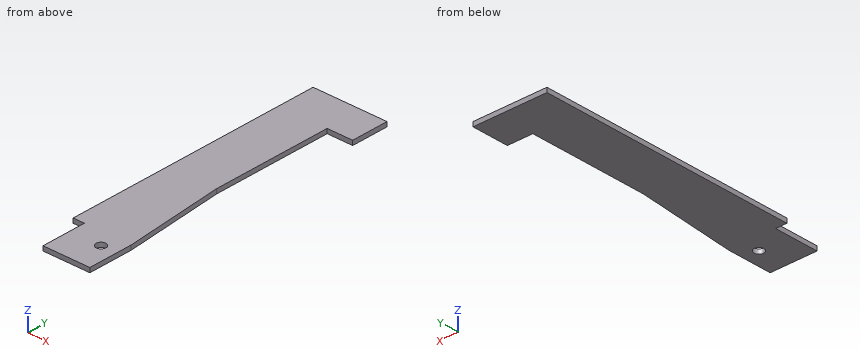
```python
from build123d import *

# Parameters (mm, degrees)
EXTRUDE_2_DEPTH     = 1
SKETCH_1_5_W        = 5.5
SKETCH_1_5_H        = 10
SKETCH_1_5_W_2      = 4.949873967
SKETCH_1_5_R        = 1.1
EXTRUDE_3_DEPTH     = 1
SKETCH_3_W          = 3
SKETCH_3_H          = 58
CUT_EXTRUDE_1_DEPTH = 10


with BuildPart() as part:
    # 草图1 → 凸台-拉伸2 (new body)
    with BuildSketch(Plane.XY):
        Polygon((-5.588804059, 13.118731113), (-5.588804059, -12.701827406), (-5.588804059, -40.201827406), (-0.088804059, -40.201827406), (5.411195941, -40.201827406), (10.361069908, -40.201827406), (8.211195941, -17.197725842), (8.211195941, 9.5), (13.911195941, 9.5), (13.911195941, 12.5), (13.911195941, 17.798172594), (-5.588804059, 17.798172594), align=None)
    extrude(amount=EXTRUDE_2_DEPTH)

    # 草图1<5> → 凸台-拉伸3 (add)
    # profile 1 of 3: a face of its own
    with BuildSketch(Plane.XY):
        Polygon((-5.588804059, 13.118731113), (-5.588804059, -12.701827406), (-5.588804059, -40.201827406), (-0.088804059, -40.201827406), (5.411195941, -40.201827406), (10.361069908, -40.201827406), (8.211195941, -17.197725842), (8.211195941, 9.5), (13.911195941, 9.5), (13.911195941, 12.5), (13.911195941, 17.798172594), (-5.588804059, 17.798172594), align=None)
    # profile 2 of 3: a face of its own
    with BuildSketch(Plane.XY):
        with Locations((2.661195941, -45.201827406)):
            Rectangle(SKETCH_1_5_W, SKETCH_1_5_H)
    # profile 3 of 3: a face of its own
    with BuildSketch(Plane.XY):
        with Locations((7.886132925, -45.201827406)):
            Rectangle(SKETCH_1_5_W_2, SKETCH_1_5_H)
        with Locations((6.861069908, -43.701827406)):
            Circle(SKETCH_1_5_R, mode=Mode.SUBTRACT)
    extrude(amount=EXTRUDE_3_DEPTH)

    # 草图3 → 切除-拉伸1 (cut)
    with BuildSketch(Plane.XY.offset(1)):
        with Locations((-4.088804059, -11.201827406)):
            Rectangle(SKETCH_3_W, SKETCH_3_H)
    extrude(amount=-CUT_EXTRUDE_1_DEPTH, mode=Mode.SUBTRACT)


solid = part.part
```
Design review of the part built by this model. Coordinates are the model's own, in mm. Round coordinates to 2 decimals unless told otherwise and drop trailing zeros. Write each loop counter-clockwise with the first axis right and the second up, starting at its lowest first coordinate (ties: lowest second). Pieces come first, ordered by that corner, then holes. Notation, with made-up numbers: (78.5, 67.5) -> (106.5, 67.5) arc R25 ccw to (106.5, 93.5) -> close; hole circle Ø4 at (8.25, 49). An arc over 180 degrees is marked (long way). Answer in a Markdown table with one row per item.
Q1. Take a section at C-C, the plane y = -41.5. State the section outline as (x, z) points.
The answers:
| item | result |
|---|---|
| outline | (-0.09, 0) -> (10.36, 0) -> (10.36, 1) -> (-0.09, 1) -> close |
Q2. Clearance check with flat-ended pins moving along their axes: pin 1 Ø0.5 at (y, z) = (-1.5, 0.5) entering from +X; pin 2 Ø1.8 at (x, y) = (6.86, -43.7) entering from -Z. State where each tip first meets the part, or that it passes through.
The answers:
| item | result |
|---|---|
| pin 1 | x = 8.21 |
| pin 2 | through |
Q3. To check wall thickness, follow L1, parallel to Y at x = -0.5, z = 0.65; L2, parallel to X at y = 7, z = 0.25; L3, parallel to X at y = -47, z = 0.75. State the ranges of each line that lie inside material, in increasing order. Write a range as [from, to].
The answers:
| item | result |
|---|---|
| L1 | [-40.2, 17.8] |
| L2 | [-2.59, 8.21] |
| L3 | [-0.09, 10.36] |
Q4. Take a section at B-B, the plane z = 0.3. State the section outline as (x, y) points, then the cut area to 3 significant figures.
The answers:
| item | result |
|---|---|
| outline | (-2.59, -40.2) -> (-0.09, -40.2) -> (-0.09, -50.2) -> (10.36, -50.2) -> (10.36, -40.2) -> (8.21, -17.2) -> (8.21, 9.5) -> (13.91, 9.5) -> (13.91, 17.8) -> (-2.59, 17.8) -> close; hole circle Ø2.2 at (6.86, -43.7) |
| area | 799 mm² |
Q5. Take a section at D-D, the plane y = -6. State the section outline as (x, z) points.
The answers:
| item | result |
|---|---|
| outline | (-2.59, 0) -> (8.21, 0) -> (8.21, 1) -> (-2.59, 1) -> close |
Q6. Take a section at A-A, the plane x = 6.75. State the section outline as (y, z) points.
The answers:
| item | result |
|---|---|
| outline | (-50.2, 0) -> (-44.8, 0) -> (-44.8, 1) -> (-50.2, 1) -> close; (-42.61, 0) -> (17.8, 0) -> (17.8, 1) -> (-42.61, 1) -> close |
